Work out the finished part from the listing and answer in its coordinate system (mm). Round coordinates to 2 decimals unless told otherwise and drop trailing zeros. Loops run counter-clockwise (first coordinate to the right, second up) from the corner with the lowest first, then second, coordinate; pieces in that order, holes last.
```python
from build123d import *

# Parameters (mm, degrees)
SKETCH_1_W          = 75
SKETCH_1_H          = 20
EXTRUDE_1_DEPTH     = 3
SKETCH_2_R          = 1.5
SKETCH_2_R_2        = 2
CUT_EXTRUDE_1_DEPTH = 4
FILLET_1_R          = 10
FILLET_2_R          = 2


with BuildPart() as part:
    # 草图1 → 凸台-拉伸1 (new body)
    with BuildSketch(Plane.XY):
        with Locations((37.5, 10)):
            Rectangle(SKETCH_1_W, SKETCH_1_H)
    extrude(amount=EXTRUDE_1_DEPTH)

    # 草图2 → 切除-拉伸1 (cut)
    with BuildSketch(Plane.XY.offset(3)):
        with Locations((70, 15)):
            Circle(SKETCH_2_R)
        with Locations((70, 5)):
            Circle(SKETCH_2_R)
        with Locations((60, 15)):
            Circle(SKETCH_2_R)
        with Locations((60, 5)):
            Circle(SKETCH_2_R)
        with Locations((5, 10)):
            Circle(SKETCH_2_R_2)
    extrude(amount=-CUT_EXTRUDE_1_DEPTH, mode=Mode.SUBTRACT)

    # 圆角1
    fillet_1_edges = [part.edges().sort_by_distance(p)[0] for p in [
        (0, 0, 1.5),
        (0, 20, 1.5),
    ]]
    fillet(fillet_1_edges, radius=FILLET_1_R - 0.0001)  # a hair under: the kernel refuses the full size

    # 圆角2
    fillet_2_edges = [part.edges().sort_by_distance(p)[0] for p in [
        (75, 20, 1.5),
        (75, 0, 1.5),
    ]]
    fillet(fillet_2_edges, radius=FILLET_2_R)


solid = part.part
```
1. Find section A-A (x = 60). Write down the section's boundary in (y, z).
Answer key:
outline: (0, 0) - (3.5, 0) - (3.5, 3) - (0, 3) - close; (6.5, 0) - (13.5, 0) - (13.5, 3) - (6.5, 3) - close; (16.5, 0) - (20, 0) - (20, 3) - (16.5, 3) - close
2. Find section D-D (y = 5). Write down the section's boundary in (x, z), then the cut area to 3 significant figures.
Answer key:
outline: (1.34, 0) - (58.5, 0) - (58.5, 3) - (1.34, 3) - close; (61.5, 0) - (68.5, 0) - (68.5, 3) - (61.5, 3) - close; (71.5, 0) - (75, 0) - (75, 3) - (71.5, 3) - close
area: 203 mm2
3. Find section B-B (z = 2.55). Give the number of separate pieces and of enclosed holes in the cut face, then the cut area to 3 significant figures.
Answer key:
separate pieces: 1
enclosed holes: 5
area: 1,410 mm2
4. Given pin 1 (2.5 mm diameter, centred on x = 60, y = 5, fed in from +Z), flat-ended and moving along its own axis, determine where the tip first touches the part or whether it passes through.
Answer key:
pin 1: passes through
5. Determine the mould class of faces 1 (the face through (3.526, 11.352, 1.521)), 2 (the face through (41, 0, 1)), 3 (the face through (74.4, 19.43, 1.52)), 4 (the face through (71.43, 5.45, 1.52)) for opening direction X: +X half, -X half, draft (parallel to the pull), parting line (faces both ways), or undercut.
Answer key:
face 1: undercut
face 2: draft
face 3: +X half
face 4: undercut
6. Find section C-C (y = 11). Write down the section's boundary in (x, z).
Answer key:
outline: (0.05, 0) - (3.27, 0) - (3.27, 3) - (0.05, 3) - close; (6.73, 0) - (75, 0) - (75, 3) - (6.73, 3) - close
7. Consider probe 1 along Y at (x, z) = (70, 2.2); probe 2 along X at (y, z) = (10.25, 1.4); probe 3 along X at (y, z) = (4, 1.15). Determine where each line is inside the solid, lowest interval first.
Answer key:
probe 1: y = 0 to 3.5, 6.5 to 13.5, 16.5 to 20
probe 2: x = 0 to 3.02, 6.98 to 75
probe 3: x = 2 to 58.88, 61.12 to 68.88, 71.12 to 75
